from build123d import *

# Parameters (mm, degrees)
F0_R     = 42
F0_R_2   = 24
F1_DEPTH = 1


with BuildPart() as f1:
    # F0 (on Front) → F1 (new body)
    with BuildSketch(Plane.XZ):
        with Locations((-2.9635038227, 0.4932200536)):
            Circle(F0_R)
        with BuildLine():
            ThreePointArc((23.788972617, 23.0610069266), (29.2411666686, 14.199393792), (31.8473983055, 4.1265508975))
            ThreePointArc((31.8473983055, 4.1265508975), (34.3010642257, 3.2306934737), (35.3348577063, 0.8318795978))
            ThreePointArc((35.3348577063, 0.8318795978), (34.3241690286, -1.5448941966), (31.9111888156, -2.4658023161))
            ThreePointArc((31.9111888156, -2.4658023161), (29.5003654621, -12.5871924421), (24.2206740094, -21.5526520225))
            ThreePointArc((24.2206740094, -21.5526520225), (25.0352315525, -22.6659149008), (25.3235434051, -24.0148902537))
            ThreePointArc((25.3235434051, -24.0148902537), (23.2290393257, -27.0868244303), (19.6042830503, -26.2592563861))
            ThreePointArc((19.6042830503, -26.2592563861), (10.7426699157, -31.7114504377), (0.6698270212, -34.3176820746))
            ThreePointArc((0.6698270212, -34.3176820746), (0.6738232774, -34.4113739144), (0.6751557215, -34.5051414754))
            ThreePointArc((0.6751557215, -34.5051414754), (-2.6866895856, -37.804561903), (-5.9225261924, -34.3814725847))
            ThreePointArc((-5.9225261924, -34.3814725847), (-16.0439163184, -31.9706492312), (-25.0093758988, -26.6909577785))
            ThreePointArc((-25.0093758988, -26.6909577785), (-29.7823788162, -26.8497487699), (-29.7159802624, -22.0745668194))
            ThreePointArc((-29.7159802624, -22.0745668194), (-35.168174314, -13.2129536848), (-37.7744059509, -3.1401107903))
            ThreePointArc((-37.7744059509, -3.1401107903), (-41.2617108673, 0.1226297524), (-37.838196461, 3.4522424234))
            ThreePointArc((-37.838196461, 3.4522424234), (-35.4273731075, 13.5736325493), (-30.1476816547, 22.5390921297))
            ThreePointArc((-30.1476816547, 22.5390921297), (-30.3064726462, 27.3120950471), (-25.5312906957, 27.2456964933))
            ThreePointArc((-25.5312906957, 27.2456964933), (-16.6696775611, 32.6978905449), (-6.5968346666, 35.3041221818))
            ThreePointArc((-6.5968346666, 35.3041221818), (-3.3959309279, 38.7902491385), (-0.0021633669, 35.4915815826))
            ThreePointArc((-0.0021633669, 35.4915815826), (-0.0027429393, 35.4297362755), (-0.0044814529, 35.3679126919))
            ThreePointArc((-0.0044814529, 35.3679126919), (10.116908673, 32.9570893384), (19.0823682534, 27.6773978857))
            ThreePointArc((19.0823682534, 27.6773978857), (22.7203219768, 28.5637220129), (24.8446064847, 25.4802672814))
            ThreePointArc((24.8446064847, 25.4802672814), (24.5692063125, 24.1604961339), (23.788972617, 23.0610069266))
        make_face(mode=Mode.SUBTRACT)
        with BuildLine():
            ThreePointArc((31.9111888156, -2.4658023161), (28.7350121907, 0.7999488408), (31.8473983055, 4.1265508975))
            ThreePointArc((31.8473983055, 4.1265508975), (29.2411666686, 14.199393792), (23.788972617, 23.0610069266))
            ThreePointArc((23.788972617, 23.0610069266), (19.2338417986, 23.1243456856), (19.0823682534, 27.6773978857))
            ThreePointArc((19.0823682534, 27.6773978857), (10.116908673, 32.9570893384), (-0.0044814529, 35.3679126919))
            ThreePointArc((-0.0044814529, 35.3679126919), (-3.2702326098, 32.191736067), (-6.5968346666, 35.3041221818))
            ThreePointArc((-6.5968346666, 35.3041221818), (-16.6696775611, 32.6978905449), (-25.5312906957, 27.2456964933))
            ThreePointArc((-25.5312906957, 27.2456964933), (-24.8786168738, 26.2068262816), (-24.6505510504, 25.001330361))
            ThreePointArc((-24.6505510504, 25.001330361), (-26.6015756975, 21.9896422136), (-30.1476816547, 22.5390921297))
            ThreePointArc((-30.1476816547, 22.5390921297), (-35.4273731075, 13.5736325493), (-37.838196461, 3.4522424234))
            ThreePointArc((-37.838196461, 3.4522424234), (-35.5850915573, 2.4438718317), (-34.6618653517, 0.1545605094))
            ThreePointArc((-34.6618653517, 0.1545605094), (-35.5630514757, -2.11164601), (-37.7744059509, -3.1401107903))
            ThreePointArc((-37.7744059509, -3.1401107903), (-35.168174314, -13.2129536848), (-29.7159802624, -22.0745668194))
            ThreePointArc((-29.7159802624, -22.0745668194), (-26.1518429826, -21.4692273463), (-24.17161413, -24.4938271741))
            ThreePointArc((-24.17161413, -24.4938271741), (-24.3881593985, -25.6695426662), (-25.0093758988, -26.6909577785))
            ThreePointArc((-25.0093758988, -26.6909577785), (-16.0439163184, -31.9706492312), (-5.9225261924, -34.3814725847))
            ThreePointArc((-5.9225261924, -34.3814725847), (-2.6567750355, -31.2052959598), (0.6698270212, -34.3176820746))
            ThreePointArc((0.6698270212, -34.3176820746), (10.7426699157, -31.7114504377), (19.6042830503, -26.2592563861))
            ThreePointArc((19.6042830503, -26.2592563861), (19.6676218093, -21.7041255676), (24.2206740094, -21.5526520225))
            ThreePointArc((24.2206740094, -21.5526520225), (29.5003654621, -12.5871924421), (31.9111888156, -2.4658023161))
        make_face()
        with Locations((-2.9635038227, 0.4932200536)):
            Circle(F0_R_2, mode=Mode.SUBTRACT)
    extrude(amount=F1_DEPTH)


solid = f1.part
Model file for the job. Use its own axes, mm. Coordinates: 2 decimals unless noted, no trailing zeros. Order: outer loops, then holes, each group sorted by start corner. A loop starts at its lowest first (then second) coordinate and runs counter-clockwise, first axis right, second up. Notation, with made-up numbers: (9, 14) -> (49, 14) arc R23 ccw to (49, 40) -> close; hole circle Ø2 at (79.25, 52). An arc over 180 degrees is marked (long way). Return JSON: item names as keys, results as strings. Group by question number.
Item 1: Saw through at A-A on z = -11. Write the cut outline in (x, y).
Item 2: Saw through at B-B on x = -28. Write the cut outline in (y, z).
Item 3: Wall check: line 1 along X through (y, z) = (-0.4, 28); line 2 along X through (y, z) = (-0.7, -0.5); line 3 along X through (y, z) = (-0.75, 25). Give the ranges that are in metal, low to high. Write a range as [from, to].
Item 4: Saw through at D-D on y = -0.55. State how many separate pieces and enclosed holes the cut face has, then the cut area to 3 significant figures.
Item 5: Pull direction X, two halves, no side cores. Call faces 1 (the cylindrical face through (37.1, -0.5, 13.1)), 2 (the cylindrical face through (-6.09, -0.49, 24.29)), 3 (the flat face through (15, -1, -18)): pulls with the +X half, pulls with the -X half, needs draft (parallel to the pull), parting line crosses it, or undercut.
Item 6: Saw through at C-C on x = -4.5. Write the cut outline in (y, z), then the cut area to 3 significant figures.
Values found:
{
 "1": {"outline": "(-43.36, -1) -> (-24.03, -1) -> (-24.03, 0) -> (-43.36, 0) -> close; (18.11, -1) -> (37.43, -1) -> (37.43, 0) -> (18.11, 0) -> close"},
 "2": {"outline": "(-1, -33.23) -> (0, -33.23) -> (0, -27.75) -> (-1, -27.75) -> close; (-1, -21.24) -> (0, -21.24) -> (0, 21.7) -> (-1, 21.7) -> close; (-1, 28.3) -> (0, 28.3) -> (0, 34.22) -> (-1, 34.22) -> close"},
 "3": {"line 1": "x = [-34.7, -29.33], [-26.57, 19.41], [23.68, 28.78]", "line 2": "x = [-44.95, -41.2], [-34.73, -26.94], [21.02, 29.02], [35.05, 39.02]", "line 3": "x = [-37.07, -31.25], [-24.65, 18.28], [24.81, 31.15]"},
 "4": {"separate pieces": "1", "enclosed holes": "9", "area": "3,460 mm2"},
 "5": {"face 1": "parting line crosses it", "face 2": "undercut", "face 3": "needs draft"},
 "6": {"outline": "(-1, -41.48) -> (0, -41.48) -> (0, -37.22) -> (-1, -37.22) -> close; (-1, -31.79) -> (0, -31.79) -> (0, -23.46) -> (-1, -23.46) -> close; (-1, 24.44) -> (0, 24.44) -> (0, 32.42) -> (-1, 32.42) -> close; (-1, 38.57) -> (0, 38.57) -> (0, 42.47) -> (-1, 42.47) -> close", "area": "24.5 mm2"}
}
